Work out the finished part from the listing and answer in its coordinate system (mm). Face numbers are marked on the shaded views. A direction names the side the tool comes from. Round coordinates to 2 decimals unless told otherwise and drop trailing zeros. Write each loop counter-clockwise with the first axis right and the second up, starting at its lowest first coordinate (ties: lowest second). Pieces come first, ordered by that corner, then holes. Notation, with made-up numbers: M 60,16.5 L 118,16.5 A25 cw 118,49.5 Z; hole C 27,18 d11. An arc over 180 degrees is marked long. One line per item, written item: value. Start each with the question number.
Q1. Consider probe 1 along Y at (x, z) = (7.5, -1.45); probe 2 along Y at (x, z) = (6.75, -3.4); probe 3 along X at (y, z) = (152.5, -0.45). Determine where each line is inside the solid, lowest interval first.
Q2. Find section A-A (y = 7.5). Write down the section's boundary in (x, z).
Q3. Given pin 1 Ø4.5 at (x, y) = (6, 131) entering from -Z; pin 2 Ø1.4 at (x, y) = (5, 108) entering from -Z; pin 3 Ø2.5 at (y, z) = (51.5, -4.5) entering from +X; pin 4 Ø1 at (x, z) = (10.5, -1) entering from -Y, each flat-ended and moving along its own axis, determine where each tip first touches the part or whether it passes through.
Q4. A tool of negligible diameter and unlimited length cuts with its end or side. For the marked faces 1, 2 and 3, from which of +Z, -Z, +X, -X, +Y, -Y can it reach the whole face along a straight path? Write none if from no direction.
Q5. Find section B-B (x = 11.5). Write down the section's boundary in (y, z), and give its area (3 significant figures).
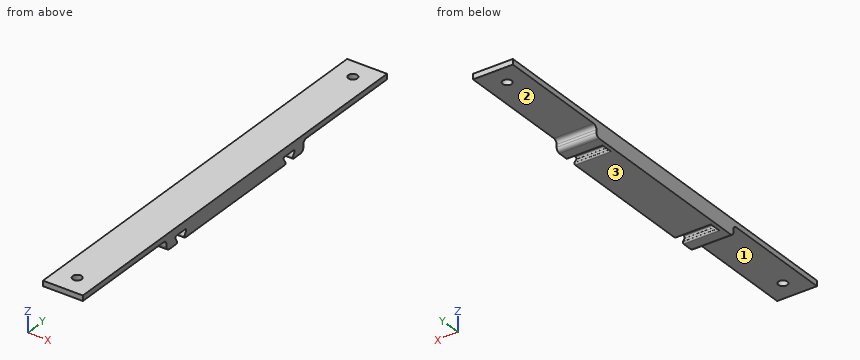
from build123d import *

# Parameters (mm, degrees)
SKETCH_1_W          = 15
SKETCH_1_H          = 160
EXTRUDE_1_DEPTH     = 2
SKETCH_4_W          = 6
SKETCH_4_H          = 15
EXTRUDE_2_DEPTH     = 15
FILLET_3_R          = 1.5
HOLE_WIZARD_M31_D   = 3.4
CUT_EXTRUDE_2_DEPTH = 13.5
FILLET_4_R          = 0.5
SKETCH_8_W          = 6
SKETCH_8_H          = 45
EXTRUDE_3_DEPTH     = 15


with BuildPart() as part:
    # Эскиз1 → Бобышка-Вытянуть1 (new body)
    with BuildSketch(Plane.XY):
        with Locations((7.5, 80)):
            Rectangle(SKETCH_1_W, SKETCH_1_H)
    extrude(amount=-EXTRUDE_1_DEPTH)

    # Эскиз4 → Бобышка-Вытянуть2 (add)
    with BuildSketch(Plane(origin=(15, 0, 0), x_dir=(0, 0, -1), z_dir=(1, 0, 0))):
        with Locations((3, 108.5)):
            Rectangle(SKETCH_4_W, SKETCH_4_H)
        with Locations((3, 51.5)):
            Rectangle(SKETCH_4_W, SKETCH_4_H)
    extrude(amount=-EXTRUDE_2_DEPTH)

    # Скругление3
    fillet_3_edges = [part.edges().sort_by_distance(p)[0] for p in [
        (7.5, 101, -6),
        (7.5, 101, -2),
        (7.5, 116, -6),
        (7.5, 116, -2),
        (7.5, 44, -6),
        (7.5, 44, -2),
        (7.5, 59, -6),
        (7.5, 59, -2),
    ]]
    fillet(fillet_3_edges, radius=FILLET_3_R)

    # Отверстие с зазором M31 (through all)
    with Locations(Plane(origin=(0, 0, -2), x_dir=(-1, 0, 0), z_dir=(0, 0, -1))):
        with Locations((-7.5, 152.5), (-7.5, 7.5)):
            Hole(HOLE_WIZARD_M31_D / 2)

    # Эскиз3 → Вырез-Вытянуть2 (cut)
    with BuildSketch(Plane(origin=(15, 0, 0), x_dir=(0, 0, -1), z_dir=(1, 0, 0))):
        Polygon((6, 110), (3, 111.732050808), (3, 105.267949192), (6, 107), align=None)
        Polygon((6, 53), (3, 54.732050808), (3, 48.267949192), (6, 50), align=None)
    extrude(amount=-CUT_EXTRUDE_2_DEPTH, mode=Mode.SUBTRACT)

    # Скругление4
    fillet_4_edges = [part.edges().sort_by_distance(p)[0] for p in [
        (8.25, 110, -6),
        (8.25, 107, -6),
        (8.25, 105.267949192, -3),
        (8.25, 111.732050808, -3),
        (8.25, 53, -6),
        (8.25, 50, -6),
        (8.25, 48.267949192, -3),
        (8.25, 54.732050808, -3),
    ]]
    fillet(fillet_4_edges, radius=FILLET_4_R)

    # Эскиз8 → Бобышка-Вытянуть3 (add)
    with BuildSketch(Plane(origin=(15, 0, 0), x_dir=(0, 0, -1), z_dir=(1, 0, 0))):
        with Locations((3, 80)):
            Rectangle(SKETCH_8_W, SKETCH_8_H)
    extrude(amount=-EXTRUDE_3_DEPTH)


solid = part.part
The answers:
1. probe 1: 0 to 5.8, 9.2 to 150.8, 154.2 to 160
1. probe 2: 44 to 48.64, 54.36 to 105.64, 111.36 to 116
1. probe 3: 0 to 5.8, 9.2 to 15
2. outline: M 0,-2 L 5.8,-2 L 5.8,0 L 0,0 Z; M 9.2,-2 L 15,-2 L 15,0 L 9.2,0 Z
3. pin 1: z = -2
3. pin 2: z = -3
3. pin 3: x = 1.5
3. pin 4: y = 0
4. face 1: -Z, +X, -X, -Y
4. face 2: -Z, +X, -X, +Y
4. face 3: -Z, +X, -X, +Y, -Y
5. outline: M 0,-2 L 42.5,-2 A1.5 cw 44,-3.5 L 44,-4.5 A1.5 ccw 45.5,-6 L 49.13,-6 A0.5 ccw 49.57,-5.25 L 48.7,-3.75 A0.5 cw 49.13,-3 L 53.87,-3 A0.5 cw 54.3,-3.75 L 53.43,-5.25 A0.5 ccw 53.87,-6 L 106.13,-6 A0.5 ccw 106.57,-5.25 L 105.7,-3.75 A0.5 cw 106.13,-3 L 110.87,-3 A0.5 cw 111.3,-3.75 L 110.43,-5.25 A0.5 ccw 110.87,-6 L 114.5,-6 A1.5 ccw 116,-4.5 L 116,-3.5 A1.5 cw 117.5,-2 L 160,-2 L 160,0 L 0,0 Z
5. area: 580 mm2
